Part model, mm, in its own coordinate system. A direction names the side the tool comes from. Give positions to 0.01 mm unless a question says otherwise; leave off trailing zeros. Order: outer loops, then holes, each group sorted by start corner. A loop starts at its lowest first (then second) coordinate and runs counter-clockwise, first axis right, second up. Notation, with made-up numbers: (-36, -22.75) - (-7, -22.75) arc R22 cw to (-7, 2.25) - close; hole circle Ø11 at (-25, 33). An arc over 180 degrees is marked (long way). One line per item, written item: value.
```python
from build123d import *

# Parameters (mm, degrees)
SKETCH2_W = 2
SKETCH2_H = 6


with BuildPart() as part:
    # Sweep1: sweep along a path in Sketch1
    with BuildLine(Plane(origin=(0, 0, 0), x_dir=(0, 0, -1), z_dir=(1, 0, 0))) as sweep1_path:
        ThreePointArc((0, 117), (-27.281180678, 96.066413802), (-14.121778265, 64.296806022))
        ThreePointArc((-14.121778265, 64.296806022), (13.053249492, 37.121778265), (23, 0))
    # Sketch2 → Sweep1 (sweep)
    with BuildSketch(Plane(origin=(0, 0, 0), x_dir=(1, 0, 0), z_dir=(0, 1, 0))):
        with Locations((1, 25.934217786)):
            Rectangle(SKETCH2_W, SKETCH2_H)
    sweep(path=sweep1_path.line)


solid = part.part
```
1) Cut at D-D, the plane z = -8.5. Give the cut face in (x, y).
Outcome:
outline: (0, 43.97) - (2, 43.97) - (2, 53.47) - (0, 53.47) - close
2) Cut at B-B, the plane x = 0.55. Give the cut face in (y, z), then the cut area to 3 significant figures.
Outcome:
outline: (0, -28.93) arc R80.18 ccw to (69.44, 11.15) arc R22.31 cw to (111.07, 0) - (117.07, 0) arc R28.31 ccw to (64.24, 14.15) arc R74.18 cw to (0, -22.93) - close
area: 882 mm^2
3) Which spindle directions (+Z, -Z, +X, -X, +Y, -Y) get a long thin tool onto all of the face, cutting with end or side? Do faces 1 (the flat face through (2, 62, 1)), 2 (the flat face through (1, 114, 0)), 3 (the cylindrical face through (0.986, 40.597, -17.897)). Say none if no direction does.
Outcome:
face 1: +Z, -Z, +X, +Y, -Y
face 2: -Z, +X, -X, +Y
face 3: -Z, +X, -X
4) Cut at C-C, the plane y = 53. Give the cut face in (x, z), then the cut area to 3 significant figures.
Outcome:
outline: (0, -8.92) - (2, -8.92) - (2, -0.65) - (0, -0.65) - close
area: 16.5 mm^2
5) Cut at A-A, the plane z = 7.5. Give the cut face in (x, y), then the cut area to 3 significant figures.
Outcome:
outline: (0, 59.91) - (2, 59.91) - (2, 67.19) - (0, 67.19) - close; (0, 109.77) - (2, 109.77) - (2, 116.05) - (0, 116.05) - close
area: 27.1 mm^2
6) Pin check, flat tips, straight feed: pin 1 (1 mm diameter, centred on x = 0.5, y = 100, fed in from -Z); pin 2 (2 mm diameter, centred on y = 36, z = -12, fed in from +X). Stop position of each tip, or through.
Outcome:
pin 1: stops at z = 18.97
pin 2: passes through
7) Drill centre lines: line 1 along Y through (x, z) = (1.9, 7); line 2 along Y through (x, z) = (1.3, 12); line 3 along Y through (x, z) = (0.3, -7.5). Where is each one in solid material? Low to high. Write a range as from..to.
Outcome:
line 1: y = 59.54..66.87, 109.94..116.19
line 2: y = 62.95..69.95, 107.56..114.4
line 3: y = 45.29..54.57
